Autodesk Inventor part; units mm, degrees
sketch "Sketch1" plane through (0, 0, 0) normal (0, 1, 0) x (-1, 0, 0)
  line L0 (95.25, -164.9778) -> (-95.25, -164.9778)
  line L1 (87.9177, -152.2778) -> (-87.9177, -152.2778)
  line L2 (95.25, -164.9778) -> (87.9177, -152.2778)
  line L3 (-95.25, -164.9778) -> (-87.9177, -152.2778)
  point P0 (0, 0)
  point P1 (0, 0)
  point P2 (0, 0)
  dimension "d0" = 190.5
  dimension "d1" = 12.7
  dimension "d3" = 120
  dimension "d4" = 0
extrude "Extrusion1" add sketch "Sketch1" along normal blind 381
sketch "Sketch2" plane through (95.25, 0, -164.9778) normal (0, 0, -1) x (-1, 0, 0)
  line L0 (25.4, 254) -> (165.1, 254)
  line L1 (165.1, 254) -> (165.1, 25.4)
  line L2 (165.1, 25.4) -> (25.4, 25.4)
  line L3 (25.4, 25.4) -> (25.4, 254)
  line L4 (0, 0) -> (0, 381)
  point P0 (95.25, 0)
  dimension "d7" = 139.7
  dimension "d8" = 25.4
  dimension "d9" = 25.4
  dimension "d10" = 228.6
extrude "Extrusion2" cut sketch "Sketch2" against normal up to next
properties part number "side_w_door"
Could you check a few things on this model? Use its own coordinates, in mm. A direction names the side the tool comes from. Give positions to 0.01 mm unless a question says otherwise; leave off trailing zeros. Order: outer loops, then holes, each group sorted by start corner. A loop starts at its lowest first (then second) coordinate and runs counter-clockwise, first axis right, second up.
1. We'd pull the mould along X, two halves only. Please class faces 1 (the flat face through (-91.635, 187.833, -158.717)), 2 (the flat face through (-1, 272, -152.278)), 3 (the flat face through (-69.85, 141, -159)), 4 (the flat face through (69.85, 138, -159)): pulls with the +X half, pulls with the -X half, needs draft (parallel to the pull), parting line crosses it, or undercut.
2. Will these pins go through, and if not, where does the flat tip stop? P1, Ø4, axis at y = 142.5, z = -158, coming from the -X side; P2, Ø3, axis at y = 105.5, z = -160.5, coming from the -X side; P3, Ø4, axis at y = 297.5, z = -161, coming from the +X side.
3. Suppose I cut it at B-B (y = 202.5). List the corners of the cut face in (x, z) for me.
4. Suppose I cut it at A-A (x = -13.5). List the corners of the cut face in (y, z) for me, plus the area to 3 significant figures.
5. Suppose I cut it at D-D (y = 320.5). List the corners of the cut face in (x, z) for me, plus the area to 3 significant figures.
6. For faces 5 (the flat face through (1, 254, -159)), 6 (the flat face through (1, 0, -159)), which set-ups out of +Z, -Z, +X, -X, +Y, -Y let a thin tool reach every point of the face, with its end or its side?
7. I need wall thicknesses on L1, parallel to Y at x = 4, z = -160.75; L2, parallel to X at y = 105, z = -157; L3, parallel to X at y = 71.5, z = -161. Which ranges of each line are inside material? Lowest first, please.
8. Suppose I cut it at C-C (z = -157). List the corners of the cut face in (x, y) for me.
Solved:
1. face 1: pulls with the -X half
1. face 2: needs draft
1. face 3: undercut
1. face 4: undercut
2. P1: stops at x = -92.38
2. P2: stops at x = -93.53
2. P3: stops at x = 94.11
3. outline: (-95.25, -164.98) - (-69.85, -164.98) - (-69.85, -152.28) - (-87.92, -152.28) - close; (69.85, -164.98) - (95.25, -164.98) - (87.92, -152.28) - (69.85, -152.28) - close
4. outline: (0, -164.98) - (25.4, -164.98) - (25.4, -152.28) - (0, -152.28) - close; (254, -164.98) - (381, -164.98) - (381, -152.28) - (254, -152.28) - close
4. area: 1,940 mm2
5. outline: (-95.25, -164.98) - (95.25, -164.98) - (87.92, -152.28) - (-87.92, -152.28) - close
5. area: 2,330 mm2
6. face 5: +Z, -Z
6. face 6: +Z, -Z, +X, -X, -Y
7. L1: y = 0 to 25.4, 254 to 381
7. L2: x = -90.64 to -69.85, 69.85 to 90.64
7. L3: x = -92.95 to -69.85, 69.85 to 92.95
8. outline: (-90.64, 0) - (90.64, 0) - (90.64, 381) - (-90.64, 381) - close; hole (-69.85, 25.4) - (69.85, 25.4) - (69.85, 254) - (-69.85, 254) - close
